```python
from build123d import *

# Parameters (mm, degrees)
EXTRUDE_1_DEPTH     = 6
SKETCH_2_R          = 2
CUT_EXTRUDE_1_DEPTH = 5


with BuildPart() as part:
    # Эскиз1 → Бобышка-Вытянуть1 (new body)
    with BuildSketch(Plane.XY):
        Polygon((0, 0), (0, 4), (6, 4), (6, 10.3), (12, 10.3), (12, 7.8), (9, 7.8), (9, 6), (12, 6), (12, 0), align=None)
    extrude(amount=EXTRUDE_1_DEPTH)

    # Эскиз2 → Вырез-Вытянуть1 (cut, through all)
    with BuildSketch(Plane(origin=(0, 4, 0), x_dir=(1, 0, 0), z_dir=(0, 1, 0))):
        with Locations((3, -3)):
            Circle(SKETCH_2_R)
    extrude(amount=-CUT_EXTRUDE_1_DEPTH, mode=Mode.SUBTRACT)


solid = part.part
```
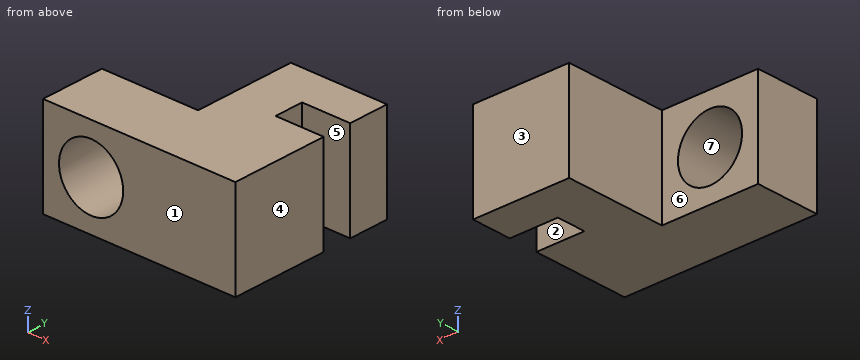
The model under review builds one solid part; all positions refer to its coordinate system, in mm. Face numbers are marked on the shaded views. A direction names the side the tool comes from. Round coordinates to 2 decimals unless told otherwise and drop trailing zeros. Write each loop counter-clockwise with the first axis right and the second up, starting at its lowest first coordinate (ties: lowest second). Pieces come first, ordered by that corner, then holes.
(1) We need section C-C on z = 1.8. Give the boundary of the cut face in (x, y).
(2) Wall thickness on L1, parallel to X at y = 2.75, z = 3; L2, parallel to Z at x = 3, y = 1.9; L3, parallel to Y at x = 11.25, z = 1.3: over which ranges is each line inside the solid? List them lowest first.
(3) Mouldability with a two-part tool opening along Y and no side actions: class the marked faces 1, 2, 3 and 4 as +Y half, -Y half, draft (parallel to the pull), parting line (faces both ways), or undercut.
(4) We need section A-A on z = 3. Give the boundary of the cut face in (x, y).
(5) Insertion check: pin 1 (3 mm diameter, centred on x = 10, y = 5.5, fed in from -Z); pin 2 (3 mm diameter, centred on x = 2, z = 1, fed in from +Y); pin 3 (3.5 mm diameter, centred on x = 3, z = 3, fed in from -Y); pin 4 (0.5 mm diameter, centred on y = 6.5, z = 4, fed in from +X). Each pin has a flat end and moves straight along its axis. Give the tip position at first contact, or say it passes through.
(6) We need section B-B on x = 3. Give the boundary of the cut face in (y, z), and give its area (3 significant figures).
(7) We need section D-D on y = 6.25. Give the boundary of the cut face in (x, z).
(8) Machinability: for the marked faces 5, 6 and 7, which of the approach directions +Z, -Z, +X, -X, +Y, -Y give a long, thin tool a straight path to every point of the face, cutting with its end or side? Answer none if there is none.
Findings below:
1. outline: (0, 0) - (1.4, 0) - (1.4, 4) - (0, 4) - close; (4.6, 0) - (12, 0) - (12, 6) - (9, 6) - (9, 7.8) - (12, 7.8) - (12, 10.3) - (6, 10.3) - (6, 4) - (4.6, 4) - close
2. L1: x = 0 to 1, 5 to 12
2. L2: z = 0 to 1, 5 to 6
2. L3: y = 0 to 6, 7.8 to 10.3
3. face 1: -Y half
3. face 2: undercut
3. face 3: +Y half
3. face 4: draft
4. outline: (0, 0) - (1, 0) - (1, 4) - (0, 4) - close; (5, 0) - (12, 0) - (12, 6) - (9, 6) - (9, 7.8) - (12, 7.8) - (12, 10.3) - (6, 10.3) - (6, 4) - (5, 4) - close
5. pin 1: stops at z = 0
5. pin 2: stops at y = 4
5. pin 3: passes through
5. pin 4: stops at x = 9
6. outline: (0, 0) - (4, 0) - (4, 1) - (0, 1) - close; (0, 5) - (4, 5) - (4, 6) - (0, 6) - close
6. area: 8.00 mm2
7. outline: (6, 0) - (9, 0) - (9, 6) - (6, 6) - close
8. face 5: +Z, -Z, +X
8. face 6: +Z, -Z, -X, +Y
8. face 7: +Y, -Y
